```python
from build123d import *

# Parameters (mm, degrees)
BOSS_EXTRUDE1_DEPTH             = 214
TAP_DRILL_FOR_M3X0_5_TAP1_D     = 4.3
TAP_DRILL_FOR_M3X0_5_TAP1_DEPTH = 6.825
TAP_DRILL_FOR_M3X0_5_TAP2_D     = 4.3
TAP_DRILL_FOR_M3X0_5_TAP2_DEPTH = 6.825


with BuildPart() as part:
    # Sketch1 → Boss-Extrude1 (new body)
    with BuildSketch(Plane.XY):
        Polygon((0, -10), (10, -10), (10, 10), (-10, 10), (-10, 0), (0, 0), align=None)
    extrude(amount=-BOSS_EXTRUDE1_DEPTH)

    # Tap Drill for M3x0.5 Tap1
    with Locations(Plane(origin=(10, 0, 0), x_dir=(0, 0, -1), z_dir=(1, 0, 0))):
        with Locations((34, 0), (64, 0), (94, 0), (124, 0), (154, 0), (184, 0)):
            Hole(TAP_DRILL_FOR_M3X0_5_TAP1_D / 2, depth=TAP_DRILL_FOR_M3X0_5_TAP1_DEPTH)

    # Tap Drill for M3x0.5 Tap2
    with Locations(Plane(origin=(0, 10, 0), x_dir=(1, 0, 0), z_dir=(0, 1, 0))):
        with Locations((0, 34), (0, 64), (0, 94), (0, 124), (0, 154), (0, 184)):
            Hole(TAP_DRILL_FOR_M3X0_5_TAP2_D / 2, depth=TAP_DRILL_FOR_M3X0_5_TAP2_DEPTH)


solid = part.part
```
Check sheet for the modelled part. Datum: model origin and axes. Units: mm. A direction names the side the tool comes from. Coordinates: 2 decimals unless noted, no trailing zeros. Order: outer loops, then holes, each group sorted by start corner. A loop starts at its lowest first (then second) coordinate and runs counter-clockwise, first axis right, second up. Notation, with made-up numbers: M 21,7.25 L 71,7.25 A15 cw 71,15.25 Z; hole C 78,42 d11. An arc over 180 degrees is marked long. Write each question's results on one line, items separated by ' | '. Start each with the question number.
1. Cross-section at A-A on x = 5.5. Record the cut outline in (y, z).
2. Go/stop test with flat-tipped pins: P1, Ø2, axis at y = 0, z = -94.5, coming from the +X side (3 decimals); P2, Ø3.5, axis at x = 0, z = -64, coming from the +Y side (3 decimals). Record where each tip stops, or that it passes through.
3. Cross-section at B-B on z = -64. Record the cut outline in (x, y) (3 decimals).
4. Cross-section at C-C on y = -7.5. Record the cut outline in (x, z).
5. Access from +Z, -Z, +X, -X, +Y, -Y to the whole of each face (thin tool, end or side, straight path). Record for faces 4 (the face through (10, 0, -106)), 5 (the face through (6.54, 0.09, -96.15)), 6 (the face through (-5, 0, -106)), 7 (the face through (0, 10, -106)), 8 (the face through (0.47, 6.54, -121.9)).
6. Material ranges on probe 1 along X at (y, z) = (5, -64); probe 2 along X at (y, z) = (-1.5, -16.5), recorded low to high.
7. Mould release check, pull along Z, two halves, no side actions. Record for faces 1 (the face through (3.175, 0, -64)), 2 (the face through (0, -5, -106)), 3 (the face through (2, 2, 0)): +Z half, -Z half, draft (parallel to the pull), parting line (faces both ways), or undercut.
Checks:
1) outline: M -10,-214 L 10,-214 L 10,0 L -10,0 Z; hole C 0,-184 d4.3; hole C 0,-154 d4.3; hole C 0,-124 d4.3; hole C 0,-94 d4.3; hole C 0,-64 d4.3; hole C 0,-34 d4.3
2) P1: stops at x = 3.175 | P2: stops at y = 3.175
3) outline: M -10,0 L 0,0 L 0,-10 L 10,-10 L 10,-2.15 L 3.175,-2.15 L 3.175,2.15 L 10,2.15 L 10,10 L 2.15,10 L 2.15,3.175 L -2.15,3.175 L -2.15,10 L -10,10 Z
4) outline: M 0,-214 L 10,-214 L 10,0 L 0,0 Z
5) face 4: +Z, -Z, +X, +Y, -Y | face 5: +X | face 6: +Z, -Z, -X, -Y | face 7: +Z, -Z, +X, -X, +Y | face 8: +Y
6) probe 1: x = -10 to -2.15, 2.15 to 10 | probe 2: x = 0 to 10
7) face 1: undercut | face 2: draft | face 3: +Z half
